The listing builds one solid part. Answer for the finished solid, in the listing's coordinates (mm). A direction names the side the tool comes from. Give positions to 0.01 mm unless a question says otherwise; leave off trailing zeros. Write each loop counter-clockwise with the first axis right and the second up, starting at its lowest first coordinate (ties: lowest second). Pieces come first, ordered by that corner, then holes. Notation, with made-up numbers: M 51,-1.5 L 68,-1.5 A14 cw 68,19.5 Z; hole C 8.25,44 d4. An arc over 180 degrees is marked long. Return JSON: item names as keys, results as strings.
from build123d import *

# Parameters (mm, degrees)
SKETCH1_W           = 35
SKETCH1_H           = 8
BOSS_EXTRUDE1_DEPTH = 12.5
CUT_EXTRUDE1_REACH  = 24.946
SKETCH2_R           = 7.5
FILLET1_R           = 10
SKETCH3_R           = 8
CUT_EXTRUDE2_DEPTH  = 2.75
SKETCH4_R           = 1.6
CUT_EXTRUDE3_DEPTH  = 22.874642854
SKETCH5_R           = 2.5
CUT_EXTRUDE4_DEPTH  = 20.455076607


with BuildPart() as part:
    # Sketch1 → Boss-Extrude1 (new body)
    with BuildSketch(Plane(origin=(0, 0, 0), x_dir=(1, 0, 0), z_dir=(0, 1, 0))):
        Rectangle(SKETCH1_W, SKETCH1_H)
    extrude(amount=BOSS_EXTRUDE1_DEPTH)

    # Sketch2 → Cut-Extrude1 (cut, up to next)
    with BuildSketch(Plane.XY.offset(4), mode=Mode.PRIVATE) as cut_extrude1_sk1:
        Circle(SKETCH2_R)
    cut_extrude1_tool1 = extrude(cut_extrude1_sk1.sketch, amount=-CUT_EXTRUDE1_REACH, mode=Mode.PRIVATE) & part.part
    add(cut_extrude1_tool1.solids().sort_by_distance((0, 0, 4))[0], mode=Mode.SUBTRACT)

    # Fillet1
    fillet1_edges = [part.edges().sort_by_distance(p)[0] for p in [
        (-17.5, 12.5, 0),
        (17.5, 12.5, 0),
    ]]
    fillet(fillet1_edges, radius=FILLET1_R)

    # Sketch3 → Cut-Extrude2 (cut, symmetric)
    with BuildSketch(Plane.XY):
        Circle(SKETCH3_R)
    extrude(amount=CUT_EXTRUDE2_DEPTH, both=True, mode=Mode.SUBTRACT)

    # Sketch4 → Cut-Extrude3 (cut, through all)
    with BuildSketch(Plane.XZ):
        with Locations(Location((13.5, 0, 0), (0, 0, 270))):
            Circle(SKETCH4_R)
        with Locations(Location((-13.5, 0, 0), (0, 0, 270))):
            Circle(SKETCH4_R)
    extrude(amount=-CUT_EXTRUDE3_DEPTH, mode=Mode.SUBTRACT)

    # Sketch5 → Cut-Extrude4 (cut, through all)
    with BuildSketch(Plane(origin=(0, 7.5, 0), x_dir=(-1, 0, 0), z_dir=(0, -1, 0))):
        with Locations(Location((-13.5, 0, 0), (0, 0, 90))):
            Circle(SKETCH5_R)
        with Locations(Location((13.5, 0, 0), (0, 0, 90))):
            Circle(SKETCH5_R)
    extrude(amount=-CUT_EXTRUDE4_DEPTH, mode=Mode.SUBTRACT)


solid = part.part
Item 1: Which of the six approach directions +Z, -Z, +X, -X, +Y, -Y give full straight-line access (tool end or side, diameter ignored) to faces 1 (the flat face through (0, 12.5, 0)), 2 (the cylindrical face through (0, 8, 0)), 3 (the cylindrical face through (-11, 9, 0))?
Geometry results:
{"face 1": "+Z, -Z, +X, -X, +Y", "face 2": "-Y", "face 3": "+Y"}
Item 2: Find the intervals of material crossed by line 1 (X direction, y = 4.75, z = 0); line 2 (X direction, y = 6.25, z = -0.75); line 3 (X direction, y = 6.5, z = -2.25), in increasing order.
Geometry results:
{"line 1": "x = -17.24 to -15.1, -11.9 to -6.44, 6.44 to 11.9, 15.1 to 17.24", "line 2": "x = -16.77 to -14.91, -12.09 to -4.99, 4.99 to 12.09, 14.91 to 16.77", "line 3": "x = -16.67 to -4.66, 4.66 to 16.67"}
Item 3: A cutting plane is placed at D-D, the plane x = 0. Write down the section's boundary in (y, z), plus the area to 4 significant figures.
Geometry results:
{"outline": "M 7.5,-4 L 12.5,-4 L 12.5,4 L 7.5,4 L 7.5,2.75 L 8,2.75 L 8,-2.75 L 7.5,-2.75 Z", "area": "37.25 mm2"}
Item 4: A cutting plane is placed at A-A, the plane x = 13.5. Write down the section's boundary in (y, z).
Geometry results:
{"outline": "M 0,-4 L 10.5,-4 L 10.5,-2.5 L 7.5,-2.5 L 7.5,-1.6 L 0,-1.6 Z; M 0,1.6 L 7.5,1.6 L 7.5,2.5 L 10.5,2.5 L 10.5,4 L 0,4 Z"}
Item 5: A cutting plane is placed at B-B, the plane y = 3.25. Write down the section's boundary in (x, z), plus the area to 3 significant figures.
Geometry results:
{"outline": "M -17.47,-4 L -6.76,-4 L -6.76,-2.75 L -7.31,-2.75 L -7.31,2.75 L -6.76,2.75 L -6.76,4 L -17.47,4 Z; M 6.76,-4 L 17.47,-4 L 17.47,4 L 6.76,4 L 6.76,2.75 L 7.31,2.75 L 7.31,-2.75 L 6.76,-2.75 Z; hole C -13.5,0 d3.2; hole C 13.5,0 d3.2", "area": "149 mm2"}
Item 6: Given pin 1 Ø6.5 at (x, y) = (-2.5, 5.5) entering from -Z; pin 2 Ø1.5 at (x, z) = (-1, -3) entering from -Y; pin 3 Ø4 at (y, z) = (10.5, -3) entering from +X; pin 4 Ø1.5 at (x, z) = (13.5, 1) entering from +Y, each flat-ended and moving along its own axis, determine where each tip first touches the part or whether it passes through.
Geometry results:
{"pin 1": "stops at z = -4", "pin 2": "stops at y = 7.29", "pin 3": "stops at x = 15.5", "pin 4": "stops at y = 7.5"}
Item 7: A cutting plane is placed at C-C, the plane z = 1. Write down the section's boundary in (x, y), plus the area to 3 significant figures.
Geometry results:
{"outline": "M -17.5,0 L -14.75,0 L -14.75,7.5 L -15.79,7.5 L -15.79,8.09 A10 ccw -17.5,2.5 Z; M -12.25,0 L -8,0 A8 cw 8,0 L 12.25,0 L 12.25,7.5 L 11.21,7.5 L 11.21,11.79 A10 ccw 7.5,12.5 L -7.5,12.5 A10 ccw -11.21,11.79 L -11.21,7.5 L -12.25,7.5 Z; M 14.75,0 L 17.5,0 L 17.5,2.5 A10 ccw 15.79,8.09 L 15.79,7.5 L 14.75,7.5 Z", "area": "231 mm2"}
